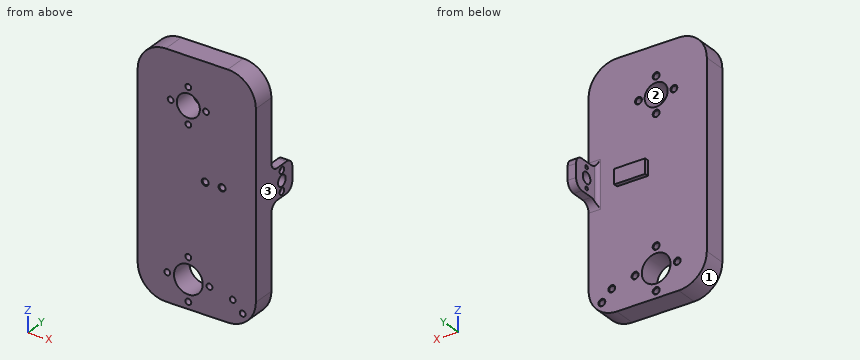
from build123d import *

# Parameters (mm, degrees)
SKETCH2_W                  = 53.34
SKETCH2_H                  = 107.950000118
SKETCH2_R                  = 5.207
SKETCH2_R_2                = 6.477
BOSS_EXTRUDE2_DEPTH        = 10.16
SKETCH14_R                 = 1.325
CUT_EXTRUDE5_DEPTH         = 93.555367213
CHAMFER2_SIZE              = 0.254
F_2_6_2_6_DIAMETER_HOLE1_D = 2.6
SKETCH5_W                  = 13.716
SKETCH5_H                  = 13.716
SKETCH5_R                  = 0.85
SKETCH5_R_2                = 2.5
BOSS_EXTRUDE3_DEPTH        = 3.81
SKETCH6_R                  = 1.5
CUT_EXTRUDE1_DEPTH         = 1.5
SKETCH7_W                  = 14.000233874
SKETCH7_H                  = 6.633249624
BOSS_EXTRUDE4_DEPTH        = 1.8542
FILLET1_R                  = 12.7
FILLET2_R                  = 3.81
FILLET3_R                  = 1.651
SKETCH13_R                 = 1.3
CUT_EXTRUDE4_DEPTH         = 94.012897289
CHAMFER3_SIZE              = 0.254
CHAMFER1_SIZE              = 0.254
SKETCH16_R                 = 1.325
CUT_EXTRUDE6_DEPTH         = 8.255
CHAMFER4_SIZE              = 0.254


with BuildPart() as part:
    # Sketch2 → Boss-Extrude2 (new body)
    with BuildSketch(Plane(origin=(0, 0, 0), x_dir=(1, 0, 0), z_dir=(0, 1, 0))):
        with Locations((3.81, 32.824999941)):
            Rectangle(SKETCH2_W, SKETCH2_H)
        with Locations(Location((0, 0, 0), (0, 0, 270))):
            Circle(SKETCH2_R, mode=Mode.SUBTRACT)
        with Locations(Location((0, 74.1, 0), (0, 0, 270))):
            Circle(SKETCH2_R_2, mode=Mode.SUBTRACT)
    extrude(amount=BOSS_EXTRUDE2_DEPTH)

    # Sketch14 → Cut-Extrude5 (cut, through all)
    with BuildSketch(Plane(origin=(0, 10.16, 0), x_dir=(1, 0, 0), z_dir=(0, 1, 0))):
        with Locations(Location((0, 83.625, 0), (0, 0, 270))):
            Circle(SKETCH14_R)
        with Locations(Location((-9.525, 74.1, 0), (0, 0, 270))):
            Circle(SKETCH14_R)
        with Locations(Location((9.525, 74.1, 0), (0, 0, 270))):
            Circle(SKETCH14_R)
        with Locations(Location((0, 64.575, 0), (0, 0, 270))):
            Circle(SKETCH14_R)
    extrude(amount=-CUT_EXTRUDE5_DEPTH, mode=Mode.SUBTRACT)

    # Chamfer2
    chamfer2_edges = [part.edges().sort_by_distance(p)[0] for p in [
        (0, 10.16, -84.95),
        (-9.525, 10.16, -75.425),
        (9.525, 10.16, -75.425),
        (0, 10.16, -65.9),
    ]]
    chamfer(chamfer2_edges, length=CHAMFER2_SIZE)

    # Ø2.6 (2.6) Diameter Hole1 (through all)
    with Locations(Plane(origin=(0, 10.16, 0), x_dir=(1, 0, 0), z_dir=(0, 1, 0))):
        with Locations((-8, 0), (0, 8), (8, 0), (0, -8)):
            Hole(F_2_6_2_6_DIAMETER_HOLE1_D / 2)

    # Sketch5 → Boss-Extrude3 (add)
    with BuildSketch(Plane(origin=(30.48, 0, 0), x_dir=(0, 0, -1), z_dir=(1, 0, 0))):
        with Locations((30.157999882, 17.018)):
            Rectangle(SKETCH5_W, SKETCH5_H)
        with Locations((25.657999882, 17.018)):
            Circle(SKETCH5_R, mode=Mode.SUBTRACT)
        with Locations((34.657999882, 17.018)):
            Circle(SKETCH5_R, mode=Mode.SUBTRACT)
        with Locations((30.157999882, 17.018)):
            Circle(SKETCH5_R_2, mode=Mode.SUBTRACT)
    extrude(amount=-BOSS_EXTRUDE3_DEPTH)

    # Sketch6 → Cut-Extrude1 (cut)
    with BuildSketch(Plane(origin=(30.48, 0, 0), x_dir=(0, 0, -1), z_dir=(1, 0, 0))):
        with Locations((25.657999882, 17.018)):
            Circle(SKETCH6_R)
        with Locations((34.657999882, 17.018)):
            Circle(SKETCH6_R)
    extrude(amount=-CUT_EXTRUDE1_DEPTH, mode=Mode.SUBTRACT)

    # Sketch7 → Boss-Extrude4 (add)
    with BuildSketch(Plane(origin=(0, 10.16, 0), x_dir=(1, 0, 0), z_dir=(0, 1, 0))):
        with Locations((10.669883029, 30.157999882)):
            Rectangle(SKETCH7_W, SKETCH7_H)
    extrude(amount=BOSS_EXTRUDE4_DEPTH)

    # Fillet1
    fillet1_edges = [part.edges().sort_by_distance(p)[0] for p in [
        (-22.86, 5.08, -86.8),
        (30.48, 5.08, -86.8),
        (30.48, 5.08, 21.150000118),
        (-22.86, 5.08, 21.150000118),
    ]]
    fillet(fillet1_edges, radius=FILLET1_R)

    # Fillet2
    fillet2_edges = [part.edges().sort_by_distance(p)[0] for p in [
        (28.575, 10.16, -23.299999882),
        (28.575, 23.876, -23.299999882),
        (28.575, 23.876, -37.015999882),
        (28.575, 10.16, -37.015999882),
    ]]
    fillet(fillet2_edges, radius=FILLET2_R)

    # Fillet3
    fillet3_edges = [part.edges().sort_by_distance(p)[0] for p in [
        (26.67, 10.16, -30.157999882),
    ]]
    fillet(fillet3_edges, radius=FILLET3_R)

    # Sketch13 → Cut-Extrude4 (cut, through all)
    with BuildSketch(Plane(origin=(0, 10.16, 0), x_dir=(1, 0, 0), z_dir=(0, 1, 0))):
        with Locations(Location((24.515192091, 80.835192091, 0), (0, 0, 270))):
            Circle(SKETCH13_R)
        with Locations(Location((20.02506403, 76.34506403, 0), (0, 0, 270))):
            Circle(SKETCH13_R)
    extrude(amount=-CUT_EXTRUDE4_DEPTH, mode=Mode.SUBTRACT)

    # Chamfer3
    chamfer3_edges = [part.edges().sort_by_distance(p)[0] for p in [
        (24.515192091, 10.16, -82.135192091),
        (20.02506403, 10.16, -77.64506403),
    ]]
    chamfer(chamfer3_edges, length=CHAMFER3_SIZE)

    # Chamfer1
    chamfer1_edges = [part.edges().sort_by_distance(p)[0] for p in [
        (-6.7, 10.16, 0),
        (1.3, 10.16, 8),
        (9.3, 10.16, 0),
        (1.3, 10.16, -8),
    ]]
    chamfer(chamfer1_edges, length=CHAMFER1_SIZE)

    # Sketch16 → Cut-Extrude6 (cut)
    with BuildSketch(Plane.XZ):
        with Locations(Location((15.24, -30.157999882, 0), (0, 0, 270))):
            Circle(SKETCH16_R)
        with Locations(Location((7.62, -30.157999882, 0), (0, 0, 270))):
            Circle(SKETCH16_R)
    extrude(amount=-CUT_EXTRUDE6_DEPTH, mode=Mode.SUBTRACT)

    # Chamfer4
    chamfer4_edges = [part.edges().sort_by_distance(p)[0] for p in [
        (15.24, 0, -28.832999882),
        (7.62, 0, -28.832999882),
    ]]
    chamfer(chamfer4_edges, length=CHAMFER4_SIZE)


solid = part.part
Input: part model. Units: mm. Frame: model coordinates. Face numbers are marked on the shaded views. Coordinates: 2 decimals unless noted, no trailing zeros. Loops run counter-clockwise (first coordinate to the right, second up) from the corner with the lowest first, then second, coordinate; pieces in that order, holes last. Notation, with made-up numbers: (6, 53) - (36, 53) arc R32 ccw to (36, 88) - close; hole circle Ø8 at (32.25, 79.25). An arc over 180 degrees is marked (long way). Answer in a Markdown table with one row per item. Add a question column.
Item 1: Section query A-A on z = 0. Return the cut outline in (x, y).
Item 2: Contact query for flat-ended pins moving along their axis: P1, Ø5, axis at x = 21, y = 7.5, coming from the +Z side; P2, Ø3.5, axis at x = 10, z = -31, coming from the +Y side; P3, Ø3.5, axis at y = 17.018, z = -34.658, coming from the -X side. Output: stop coordinate, or through.
Item 3: Mould query, pull axis Z, two halves, no side actions, for the marked faces 1, 2 and 3. Classes: released by +Z, released by -Z, zero draft, split by the parting line, or undercut.
Item 4: Line query: line 1 along Y through (x, z) = (24, -5); line 2 along X through (y, z) = (3.5, 8); line 3 along Z through (x, y) = (28.5, 18.25). Output: solid intervals per line, ascending. Write a range as [from, to].
Item 5: Section query B-B on x = 0. State how many separate pieces and enclosed holes the cut face has, then the cut area to 3 significant figures.
Item 6: Section query D-D on x = 15.24. Return the cut outline in (y, z) (3 decimals).
Recorded:
| question | item | result |
|---|---|---|
| 1 | outline | (-22.86, 0) - (-9.3, 0) - (-9.3, 9.91) - (-9.55, 10.16) - (-22.86, 10.16) - close; (-6.7, 0) - (-5.21, 0) - (-5.21, 10.16) - (-6.45, 10.16) - (-6.7, 9.91) - close; (5.21, 0) - (6.7, 0) - (6.7, 9.91) - (6.45, 10.16) - (5.21, 10.16) - close; (9.3, 0) - (30.48, 0) - (30.48, 10.16) - (9.55, 10.16) - (9.3, 9.91) - close |
| 2 | P1 | z = 21.13 |
| 2 | P2 | y = 12.01 |
| 2 | P3 | x = 26.67 |
| 3 | face 1 | released by -Z |
| 3 | face 2 | undercut |
| 3 | face 3 | zero draft |
| 4 | line 1 | [0, 10.16] |
| 4 | line 2 | [-22.86, -1.3], [1.3, 30.48] |
| 4 | line 3 | [-37.02, -32.33], [-27.98, -23.3] |
| 5 | separate pieces | 7 |
| 5 | enclosed holes | 0 |
| 5 | area | 752 mm^2 |
| 6 | outline | (0, -86.8) - (10.16, -86.8) - (10.16, -33.475) - (12.014, -33.475) - (12.014, -26.841) - (10.16, -26.841) - (10.16, 21.15) - (0, 21.15) - (0, -28.579) - (0.254, -28.833) - (8.255, -28.833) - (8.255, -31.483) - (0.254, -31.483) - (0, -31.737) - close |
